Autodesk Inventor part; units mm, degrees
ref_plane "YZ Plane" through (0, 0, 0) normal (1, 0, 0) x (0, 1, 0)
ref_plane "XZ Plane" through (0, 0, 0) normal (0, 1, 0) x (-1, 0, 0)
ref_plane "XY Plane" through (0, 0, 0) normal (0, 0, 1) x (1, 0, 0)
sketch "Sketch2" plane through (0, 0, 0) normal (0, 1, 0) x (-1, 0, 0)
  line L0 (70, -18) -> (60, -18)
  line L1 (60, -18) -> (60, -12)
  line L2 (70, -12) -> (70, -18)
  line L3 (-70, -18.0006) -> (-60, -18.0006)
  line L4 (-60, -18.0006) -> (-60, -12.0003)
  line L5 (-70, -12.0003) -> (-70, -18.0006)
  line L6 (3, 70) -> (-3, 70)
  line L7 (-3, 70) -> (-3, 80)
  line L8 (-3, 80) -> (3, 80)
  line L9 (3, 80) -> (3, 70)
  line L10 (3, 45) -> (-3, 45)
  line L11 (-3, 45) -> (-3, 55)
  line L12 (-3, 55) -> (3, 55)
  line L13 (3, 55) -> (3, 45)
  line L14 (95, -65) -> (-95, -65)
  line L15 (-12.5, 85) -> (12.5, 85)
  line L16 (12.5, 85) -> (35.9015, 46.7742)
  line L17 (-100, -12.0003) -> (-70, -12.0003)
  line L18 (-55.4919, -12.0003) -> (-60, -12.0003)
  line L19 (55.4917, -12) -> (60, -12)
  line L20 (70, -12) -> (100, -12)
  line L21 (-100, -60) -> (-100, -12.0003)
  line L22 (100, -60) -> (100, -12)
  line L23 (35, -45) -> (-35, -45)
  line L24 (-40, -40) -> (-40, -26.409)
  line L25 (-39.2644, -23.7983) -> (-13.9141, 17.6106)
  line L26 (-9.6497, 20) -> (9.6497, 20)
  line L27 (40, -40) -> (40, -26.409)
  line L28 (39.2644, -23.7983) -> (13.9141, 17.6106)
  arc A0 (-40, -40) -> (-35, -45) centre (-35, -40) ccw
  arc A1 (-39.2644, -23.7983) -> (-40, -26.409) centre (-35, -26.409) ccw
  arc A2 (-9.6497, 20) -> (-13.9141, 17.6106) centre (-9.6497, 15) ccw
  arc A3 (13.9141, 17.6106) -> (9.6497, 20) centre (9.6497, 15) ccw
  arc A4 (40, -26.409) -> (39.2644, -23.7983) centre (35, -26.409) ccw
  arc A5 (35, -45) -> (40, -40) centre (35, -40) ccw
  line L29 (55.4917, -12) -> (35.9015, 20)
  line L30 (35.9015, 20) -> (35.9015, 46.7742)
  line L31 (-55.4919, -12.0003) -> (-35.9015, 20)
  line L32 (-35.9015, 20) -> (-35.9015, 46.7742)
  line L33 (-35.9015, 46.7742) -> (-12.5, 85)
  line L34 (0, -65) -> (0, 85) construction
  arc A6 (95, -65) -> (100, -60) centre (95, -60) ccw
  arc A7 (-100, -60) -> (-95, -65) centre (-95, -60) ccw
  point P0 (100, -65)
  point P1 (-100, -65)
  point P2 (0, 0)
  point P3 (0, 80)
  point P4 (0, 45)
  point P5 (0, 55)
  point P6 (0, 0)
  point P7 (0, 0)
  point P8 (-70, -15.4178)
  point P9 (75.3708, -12)
  point P10 (0, 0)
  point P11 (-40, -45)
  point P12 (40, -45)
  point P13 (-40, -25)
  point P14 (-12.4513, 20)
  point P15 (12.4513, 20)
  point P16 (40, -25)
  point P17 (0, 20)
  point P18 (0, -45)
  dimension "d65" = 200
  dimension "d115" = 10
  dimension "d116" = 6
  dimension "d118" = 10
  dimension "d119" = 6
  dimension "d120" = 15
  dimension "d147" = 65
  dimension "d173" = 25
  dimension "d187" = 100
  dimension "d191" = 30
  dimension "d192" = 30
  dimension "d194" = 6.0003
  dimension "d195" = 6
  dimension "d196" = 10
  dimension "d197" = 10
  dimension "d198" = 52.9997
  dimension "d199" = 53
  dimension "d204" = 150
  dimension "d213" = 20
  dimension "d214" = 20
  dimension "d218" = 65
  dimension "d219" = 40
  dimension "d220" = 5
  dimension "d233" = 148.525
  dimension "d235" = 5
  dimension "d236" = 20
  dimension "d249" = 5
extrude "Extrusion11" add sketch "Sketch2" along normal blind 3
sketch "Sketch4" plane through (0, 3, 0) normal (0, 1, 0) x (1, 0, 0)
  line L0 (-51, 38) -> (-45, 38)
  line L1 (-45, 38) -> (-45, 28)
  line L2 (-45, 28) -> (-51, 28)
  line L3 (-51, 28) -> (-51, 38)
  line L4 (95, 65) -> (-95, 65)
  line L5 (-40, 40) -> (-40, 26.409)
  line L6 (45, 38) -> (51, 38)
  line L7 (51, 38) -> (51, 28)
  line L8 (51, 28) -> (45, 28)
  line L9 (45, 28) -> (45, 38)
  line L10 (40, 40) -> (40, 26.409)
  point P0 (0, 0)
  point P1 (100, 65)
  point P2 (-100, 65)
  dimension "d237" = 6
  dimension "d238" = 27
  dimension "d239" = 10
  dimension "d240" = 5
  dimension "d241" = 6
  dimension "d242" = 10
  dimension "d243" = 5
  dimension "d244" = 27
extrude "Extrusion13" cut sketch "Sketch4" against normal through all
fillet "Fillet1" radius 15 6 edges at (12.5, 1.5, 85) (-12.5, 1.5, 85) (-35.9015, 1.5, 46.7742) (35.9015, 1.5, 46.7742) (35.9015, 1.5, 20) (-35.9015, 1.5, 20)
fillet "Fillet2" radius 5 2 edges at (55.4919, 1.5, -12.0003) (-55.4917, 1.5, -12)
properties part number "Top Plate 27100914"
The model under review builds one solid part; all positions refer to its coordinate system, in mm. A direction names the side the tool comes from. Give positions to 0.01 mm unless a question says otherwise; leave off trailing zeros. Write each loop counter-clockwise with the first axis right and the second up, starting at its lowest first coordinate (ties: lowest second). Pieces come first, ordered by that corner, then holes. Notation, with made-up numbers: M 10,84.25 L 20,84.25 A24 ccw 20,102.25 Z; hole C 32.5,88.25 d3. An arc over 180 degrees is marked long. Answer in a Markdown table with one row per item.
Item 1: For line 1 along Z through (x, y) = (-4, 1.05); line 2 along X through (y, z) = (1.2, -40); line 3 along Z through (x, y) = (86.5, 2), list the stretches that pass through material, from the lowest coordinate up.
Check sheet entries:
| item | result |
|---|---|
| line 1 | -65 to -45, 20 to 85 |
| line 2 | -100 to -40, 40 to 100 |
| line 3 | -65 to -12 |
Item 2: Add section D-D on z = 33.5. Give the boundary of the cut face in (x, y).
Check sheet entries:
| item | result |
|---|---|
| outline | M -35.9,0 L 35.9,0 L 35.9,3 L -35.9,3 Z |
Item 3: Add section C-C on y = 2.2. State how many separate pieces and enclosed holes the cut face has, plus the area to 3 significant figures.
Check sheet entries:
| item | result |
|---|---|
| separate pieces | 1 |
| enclosed holes | 5 |
| area | 13,000 mm2 |
Item 4: Add section A-A on z = -3. Give the boundary of the cut face in (x, y), plus the area to 3 significant figures.
Check sheet entries:
| item | result |
|---|---|
| outline | M -49.98,0 L -26.53,0 L -26.53,3 L -49.98,3 Z; M 26.53,0 L 49.98,0 L 49.98,3 L 26.53,3 Z |
| area | 141 mm2 |
Item 5: Add section B-B on x = 25. Give the boundary of the cut face in (y, z).
Check sheet entries:
| item | result |
|---|---|
| outline | M 0,-65 L 3,-65 L 3,-45 L 0,-45 Z; M 0,-0.5 L 3,-0.5 L 3,64.58 L 0,64.58 Z |
Item 6: For P1, Ø1, axis at y = 1.5, z = 46, coming from the +X side; P2, Ø0.5, axis at x = -59.5, y = 1.5, coming from the +Z side; P3, Ø1, axis at y = 0.5, z = 41.5, coming from the +X side, all flat-tipped, find the tip position at first contact; note any pin that passes through.
Check sheet entries:
| item | result |
|---|---|
| P1 | x = 35.61 |
| P2 | z = -12 |
| P3 | x = 35.9 |
Item 7: Tool access review of faces 1 (the face through (38, 1, -44)), 2 (the face through (-46.18, 1.48, 3.21)): name each direction out of +Z, -Z, +X, -X, +Y, -Y from which nothing blocks a thin tool from reaching the whole face with its end or side.
Check sheet entries:
| item | result |
|---|---|
| face 1 | +Y, -Y |
| face 2 | +Z, -X, +Y, -Y |
Item 8: Draft analysis for pull direction Z (two halves, no side actions). For faces 3 (the face through (-39, 1, -43)), 4 (the face through (-26.767, 1.479, -3.384)), 5 (the face through (46.18, 1.48, 3.21)), 6 (the face through (24, 3, 11)), state which applies: +Z half, -Z half, draft (parallel to the pull), parting line (faces both ways), or undercut.
Check sheet entries:
| item | result |
|---|---|
| face 3 | undercut |
| face 4 | undercut |
| face 5 | +Z half |
| face 6 | draft |
